from build123d import *

# Parameters (mm, degrees)
F0_W     = 19.8
F0_H     = 10.6
F0_R     = 1.25
F1_DEPTH = 3.2
F2_W     = 0.5
F2_H     = 3.2
F3_DEPTH = 3.5
F5_DEPTH = 2
F7_DEPTH = 4


with BuildPart() as f1:
    # F0 (on Front) → F1 (new body, symmetric)
    with BuildSketch(Plane.XZ):
        Rectangle(F0_W, F0_H)
        with Locations((-4.75, -2.4)):
            Circle(F0_R, mode=Mode.SUBTRACT)
        with Locations((4.75, -2.4)):
            Circle(F0_R, mode=Mode.SUBTRACT)
    extrude(amount=F1_DEPTH, both=True)

    # F2 (on face) → F3 (join)
    with BuildSketch(Plane(origin=(0, 0, -5.3), x_dir=(1, 0, 0), z_dir=(0, 0, -1))):
        with Locations((-8.05, 0)):
            Rectangle(F2_W, F2_H)
        with Locations((0.75, 0)):
            Rectangle(F2_W, F2_H)
        with Locations((8.05, 0)):
            Rectangle(F2_W, F2_H)
    extrude(amount=F3_DEPTH)

    # F4 (on Front) → F5 (join, symmetric)
    with BuildSketch(Plane.XZ):
        Polygon((10.80955, 10.9), (-6.9, 5.3), (-5.904972, 5.3), (10.9, 10.61396), align=None)
    extrude(amount=F5_DEPTH, both=True)

    # F6 (on face) → F7 (join, through all)
    with BuildSketch(Plane.XZ.offset(2)):
        with BuildLine():
            Line((6.518951, 9.543254), (10.80955, 10.9))
            Line((10.80955, 10.9), (9.769379, 14.189459))
            ThreePointArc((9.769379, 14.189459), (6.945706, 15.656386), (5.478779, 12.832714))
            Line((5.478779, 12.832714), (6.518951, 9.543254))
        make_face()
    extrude(amount=-F7_DEPTH)


solid = f1.part
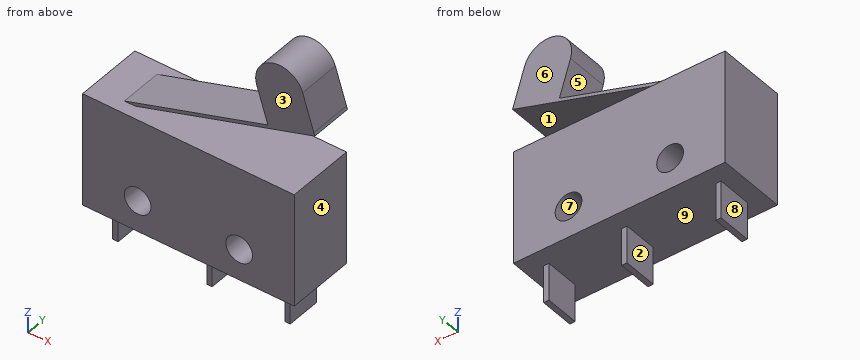
Model file for the job. Use its own axes, mm. Face numbers are marked on the shaded views. A direction names the side the tool comes from. Give positions to 0.01 mm unless a question says otherwise; leave off trailing zeros. Loops run counter-clockwise (first coordinate to the right, second up) from the corner with the lowest first, then second, coordinate; pieces in that order, holes last. Notation, with made-up numbers: (56.25, 81.25) -> (61.25, 81.25) arc R13 cw to (61.25, 92.25) -> close; hole circle Ø10 at (-10, 7). An arc over 180 degrees is marked (long way). Use a Markdown table: item, result. Add a question column.
(1) Slice it at C-C on x = 2.5. List the corners of the cut face in (y, z), and give its area (3 significant figures).
(2) Slice it at A-A on y = -0.25. List the corners of the cut face in (x, z), and give its area (3 significant figures).
(3) Mould opens along X. For the marked faces 6, 7, 8 and 9 say: +X half, -X half, draft (parallel to the pull), parting line (faces both ways), or undercut.
(4) Slice it at B-B on x = 4.75. List the corners of the cut face in (y, z), and give its area (3 significant figures).
(5) Wall check: line 1 along Z through (x, y) = (4.75, 1.5); line 2 along Z through (x, y) = (-4.75, -1.5); line 3 along Y through (x, z) = (9.5, 13.75). Give the ranges that are in metal, low to high.
(6) Slice it at D-D on z = -1.5. List the corners of the cut face in (x, y).
(7) Tool access for the marked faces 1, 2, 3, 4 and 5: list every direction of +Z, -Z, +X, -X, +Y, -Y with a clear straight run to the whole face (end or side of a thin tool).
(8) Drop flat-ended pins along their axis: pin 1 Ø1.6 at (y, z) = (0.5, -7) entering from -X; pin 2 Ø8 at (x, z) = (-1, 11) entering from -Y; pin 3 Ø1 at (y, z) = (0.5, -7.5) entering from +X. Give the stop position or say it passes through.
Filled sheet:
| question | item | result |
|---|---|---|
| 1 | outline | (-3.2, -5.3) -> (3.2, -5.3) -> (3.2, 5.3) -> (-3.2, 5.3) -> close; (-2, 7.96) -> (2, 7.96) -> (2, 8.27) -> (-2, 8.27) -> close |
| 1 | area | 69.1 mm2 |
| 2 | outline | (-9.9, -5.3) -> (-8.3, -5.3) -> (-8.3, -8.8) -> (-7.8, -8.8) -> (-7.8, -5.3) -> (0.5, -5.3) -> (0.5, -8.8) -> (1, -8.8) -> (1, -5.3) -> (7.8, -5.3) -> (7.8, -8.8) -> (8.3, -8.8) -> (8.3, -5.3) -> (9.9, -5.3) -> (9.9, 5.3) -> (-5.9, 5.3) -> (10.9, 10.61) -> (10.81, 10.9) -> (9.77, 14.19) arc R2.25 ccw to (5.48, 12.83) -> (6.52, 9.54) -> (-6.9, 5.3) -> (-9.9, 5.3) -> close; hole circle Ø2.5 at (-4.75, -2.4); hole circle Ø2.5 at (4.75, -2.4) |
| 2 | area | 234 mm2 |
| 3 | face 6 | draft |
| 3 | face 7 | undercut |
| 3 | face 8 | -X half |
| 3 | face 9 | undercut |
| 4 | outline | (-3.2, -5.3) -> (3.2, -5.3) -> (3.2, -3.65) -> (-3.2, -3.65) -> close; (-3.2, -1.15) -> (3.2, -1.15) -> (3.2, 5.3) -> (-3.2, 5.3) -> close; (-2, 8.67) -> (2, 8.67) -> (2, 8.98) -> (-2, 8.98) -> close |
| 4 | area | 53.1 mm2 |
| 5 | line 1 | -5.3 to -3.65, -1.15 to 5.3, 8.67 to 8.98 |
| 5 | line 2 | -5.3 to -3.65, -1.15 to 5.3, 5.67 to 5.98 |
| 5 | line 3 | -2 to 2 |
| 6 | outline | (-9.9, -3.2) -> (-5.62, -3.2) -> (-5.62, 3.2) -> (-9.9, 3.2) -> close; (-3.88, -3.2) -> (3.88, -3.2) -> (3.88, 3.2) -> (-3.88, 3.2) -> close; (5.62, -3.2) -> (9.9, -3.2) -> (9.9, 3.2) -> (5.62, 3.2) -> close |
| 7 | face 1 | +X, +Y, -Y |
| 7 | face 2 | -Z, +Y, -Y |
| 7 | face 3 | +Z, +X, -X, -Y |
| 7 | face 4 | -Z, +X, +Y, -Y |
| 7 | face 5 | -X, +Y, -Y |
| 8 | pin 1 | x = -8.3 |
| 8 | pin 2 | y = -2 |
| 8 | pin 3 | x = 8.3 |
